```python
from build123d import *

# Parameters (mm, degrees)
SALIENTE_EXTRUIR1_DEPTH = 400
REDONDEO1_R             = 10


with BuildPart() as part:
    # Croquis1 → Saliente-Extruir1 (new body)
    with BuildSketch(Plane(origin=(0, 0, 0), x_dir=(0, 0, -1), z_dir=(1, 0, 0))):
        with BuildLine():
            Line((0, 12.5), (15, 12.5))
            ThreePointArc((15, 12.5), (27.5, 0), (15, -12.5))
            Line((15, -12.5), (0, -12.5))
            ThreePointArc((0, -12.5), (-12.5, 0), (0, 12.5))
        make_face()
    extrude(amount=SALIENTE_EXTRUIR1_DEPTH)

    # Redondeo1
    redondeo1_edges = [part.edges().sort_by_distance(p)[0] for p in [
        (400, 0, -27.5),
        (400, 12.5, -7.5),
        (400, 0, 12.5),
        (400, -12.5, -7.5),
    ]]
    fillet(redondeo1_edges, radius=REDONDEO1_R)


solid = part.part
```
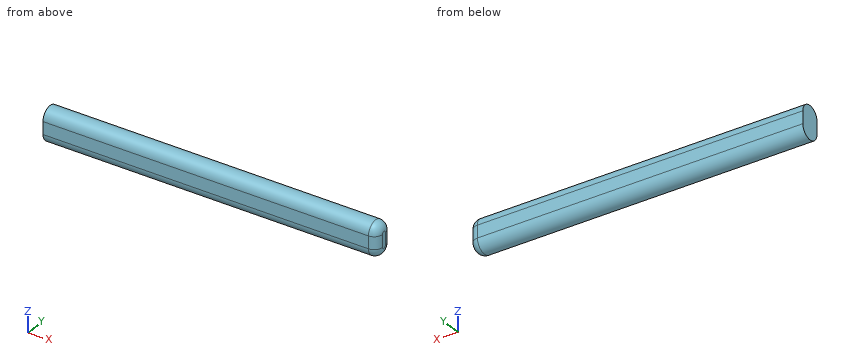
Could you check a few things on this model? Use its own coordinates, in mm. Round coordinates to 2 decimals unless told otherwise and drop trailing zeros. Loops run counter-clockwise (first coordinate to the right, second up) from the corner with the lowest first, then second, coordinate; pieces in that order, holes last. Notation, with made-up numbers: (67, 57) -> (103, 57) arc R20 cw to (103, 91) -> close; hole circle Ø9 at (-35.75, 49.5). An arc over 180 degrees is marked (long way). Put each result on its own line as item: value.
Q1. I want a section at A-A on x = 216. Write out the boundary of the cut face in (y, z), and give its area (3 significant figures).
Checks:
outline: (-12.5, -15) arc R12.5 ccw to (12.5, -15) -> (12.5, 0) arc R12.5 ccw to (-12.5, 0) -> close
area: 866 mm2
Q2. For pin 1 Ø2 at (x, z) = (104, -20.5) entering from -Y; pin 2 Ø12 at (y, z) = (9.5, -21.5) entering from +X; pin 3 Ø5 at (x, y) = (301.5, 8.5) entering from +Z, each with a flat end and sliding along its axis, tell me the tip position at first contact or that it passes through.
Checks:
pin 1: y = -11.66
pin 2: x = 399.54
pin 3: z = 10.97
Q3. Please list where these lines run through material, in increasing order: line 1 (Y direction, x = 335.5, z = 1); line 2 (Z direction, x = 292.5, y = -0.75); line 3 (X direction, y = -9, z = -3). Write a range as from..to.
Checks:
line 1: -12.46..12.46
line 2: -27.48..12.48
line 3: 0..397.6
